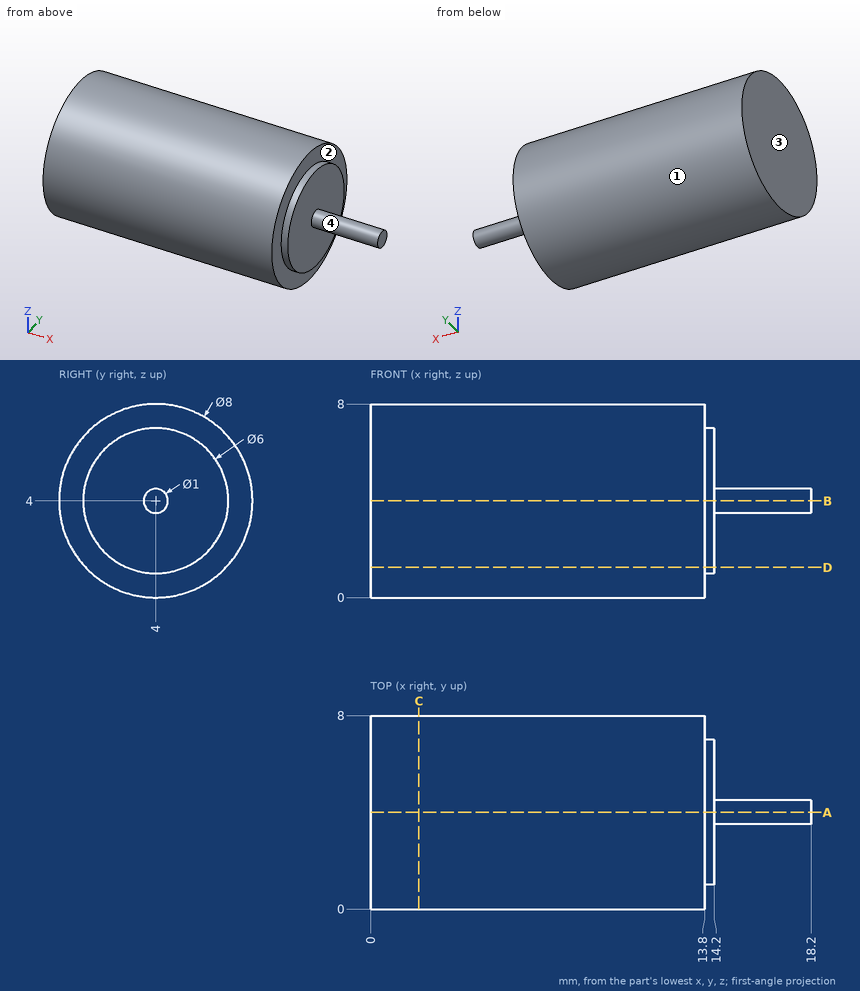
Geometry: see drawing. Coordinates: mm, zero at the bounding-box minimum. A direction names the side the tool comes from. Coordinates: 2 decimals unless noted, no trailing zeros. Loops run counter-clockwise (first coordinate to the right, second up) from the corner with the lowest first, then second, coordinate; pieces in that order, holes last. Notation, with made-up numbers: M 58.25,59 L 93.25,59 A30 ccw 93.25,87 Z; hole C -14,45.5 d8. An arc over 180 degrees is marked long. Answer in a Markdown table with one row per item.
Q1. Section D-D on z = 1.25. Return the cut outline in (x, y), plus the area to 3 significant figures.
Answers below:
| item | result |
|---|---|
| outline | M 0,1.1 L 13.8,1.1 L 13.8,2.8 L 14.2,2.8 L 14.2,5.2 L 13.8,5.2 L 13.8,6.9 L 0,6.9 Z |
| area | 81.1 mm^2 |
Q2. Section C-C on x = 2. Return the cut outline in (y, z), plus the area to 3 significant figures.
Answers below:
| item | result |
|---|---|
| outline | C 4,4 d8 |
| area | 50.3 mm^2 |
Q3. Section A-A on y = 4. Return the cut outline in (x, z).
Answers below:
| item | result |
|---|---|
| outline | M 0,0 L 13.8,0 L 13.8,1 L 14.2,1 L 14.2,3.5 L 18.2,3.5 L 18.2,4.5 L 14.2,4.5 L 14.2,7 L 13.8,7 L 13.8,8 L 0,8 Z |
Q4. Draft query along Z for the marked faces 1 and 2. Return one class per face: pulls with the +Z half, pulls with the -Z half, needs draft (parallel to the pull), parting line crosses it, or undercut.
Answers below:
| item | result |
|---|---|
| face 1 | parting line crosses it |
| face 2 | needs draft |
Q5. Ray query, probe 1 along X at (y, z) = (4.25, 3); probe 2 along X at (y, z) = (7.5, 3.5); probe 3 along Y at (x, z) = (3.25, 6.75). Return the intervals inside material, ascending. Write a range as from..to.
Answers below:
| item | result |
|---|---|
| probe 1 | x = 0..14.2 |
| probe 2 | x = 0..13.8 |
| probe 3 | y = 1.1..6.9 |
Q6. Set-up query: the marked faces 3 and 4. Return all of +Z, -Z, +X, -X, +Y, -Y with unobstructed straight access to the full face (end or side cutting, diameter ignored); none if empty.
Answers below:
| item | result |
|---|---|
| face 3 | +Z, -Z, -X, +Y, -Y |
| face 4 | +X |
Q7. First-contact query: pin 1 (1 mm diameter, centred on x = 6.5, z = 6.5, fed in from +Y); pin 2 (1 mm diameter, centred on y = 2, z = 6, fed in from +X). Flat tips, straight axial feed; report the tip coordinate or a pass-through.
Answers below:
| item | result |
|---|---|
| pin 1 | stops at y = 7.46 |
| pin 2 | stops at x = 14.2 |
